Verification items for the finished model (mm, model axes). A direction names the side the tool comes from. Coordinates: 2 decimals unless noted, no trailing zeros. Order: outer loops, then holes, each group sorted by start corner. A loop starts at its lowest first (then second) coordinate and runs counter-clockwise, first axis right, second up. Notation, with made-up numbers: M 16.5,80 L 23.5,80 A23 ccw 23.5,105 Z; hole C 41,46.5 d5. An arc over 180 degrees is marked long. Answer as a JSON object with one key per item and string values. Group by question number.
(1) Cross-section at A-A (z = 0). Enter the section's corners in (x, y), plus the area to 3 significant figures.
(2) Gauge pin test, flat ends, axial feed: pin 1 Ø1 at (y, z) = (-9, 1) entering from -X; pin 2 Ø6 at (x, y) = (4.5, -12) entering from +Z; pin 3 Ø2 at (x, y) = (-1.5, -0.5) entering from +Z. Record the tip position at first contact, or that the pin passes through.
(3) Access from +Z, -Z, +X, -X, +Y, -Y to the whole of each face (thin tool, end or side, straight path). Record for faces 4 (the face through (4.2, 0, 4.2)), 5 (the face through (-2.17, 0.99, 9.76)).
(4) Cross-section at C-C (y = -4.75). Enter the section's corners in (x, z).
(5) Mould release check, pull along Z, two halves, no side actions. Record for faces 1 (the face through (1, -18, 5)), 2 (the face through (-0.59, -7.86, -4.46)), 3 (the face through (-0.75, -8.87, 5.7)): released by +Z, released by -Z, zero draft, split by the parting line, or undercut.
(6) Material ranges on line 1 (Z direction, x = 0, y = -2.5); line 2 (Y direction, x = -7.5, z = 1.25); line 3 (X direction, y = -1, z = 0.25), recorded low to high.
(7) Cross-section at B-B (x = 0). Enter the section's corners in (y, z), plus the area to 3 significant figures.
from build123d import *

# Parameters (mm, degrees)
SKETCH_1_R          = 10
EXTRUDE_1_DEPTH     = 2
SKETCH_2_R          = 5.75
EXTRUDE_2_DEPTH     = 18
CUT_EXTRUDE_1_REACH = 22
SKETCH_3_R          = 4.5
CHAMFER_1_SIZE      = 0.25
FILLET_1_R          = 0.25


with BuildPart() as part:
    # ｽｹｯﾁ1 → ﾎﾞｽ - 押し出し1 (new body)
    with BuildSketch(Plane(origin=(0, 0, 0), x_dir=(1, 0, 0), z_dir=(0, 1, 0))):
        Circle(SKETCH_1_R)
    extrude(amount=EXTRUDE_1_DEPTH)

    # ｽｹｯﾁ2 → ﾎﾞｽ - 押し出し2 (add)
    with BuildSketch(Plane.XZ):
        Circle(SKETCH_2_R)
    extrude(amount=EXTRUDE_2_DEPTH)

    # ｽｹｯﾁ3 → ｶｯﾄ - 押し出し1 (cut, up to next)
    with BuildSketch(Plane(origin=(0, 2, 0), x_dir=(1, 0, 0), z_dir=(0, 1, 0)), mode=Mode.PRIVATE) as cut_extrude_1_sk1:
        Circle(SKETCH_3_R)
    cut_extrude_1_tool1 = extrude(cut_extrude_1_sk1.sketch, amount=-CUT_EXTRUDE_1_REACH, mode=Mode.PRIVATE) & part.part
    add(cut_extrude_1_tool1.solids().sort_by_distance((0, 2, 0))[0], mode=Mode.SUBTRACT)

    # 面取り1
    chamfer_1_edges = [part.edges().sort_by_distance(p)[0] for p in [
        (-10, 0, 0),
        (-10, 2, 0),
    ]]
    chamfer(chamfer_1_edges, length=CHAMFER_1_SIZE)

    # ﾌｨﾚｯﾄ1
    fillet_1_edges = [part.edges().sort_by_distance(p)[0] for p in [
        (-4.5, -18, 0),
        (-4.5, 2, 0),
    ]]
    fillet(fillet_1_edges, radius=FILLET_1_R)


solid = part.part
Taken from the geometry:
{
 "1": {"outline": "M -10,0.25 L -9.75,0 L -5.75,0 L -5.75,-18 L -4.75,-18 A0.25 ccw -4.5,-17.75 L -4.5,1.75 A0.25 ccw -4.75,2 L -9.75,2 L -10,1.75 Z; M 4.5,-17.75 A0.25 ccw 4.75,-18 L 5.75,-18 L 5.75,0 L 9.75,0 L 10,0.25 L 10,1.75 L 9.75,2 L 4.75,2 A0.25 ccw 4.5,1.75 Z", "area": "66.8 mm²"},
 "2": {"pin 1": "stops at x = -5.73", "pin 2": "stops at z = 5.55", "pin 3": "stops at z = 9.96"},
 "3": {"face 4": "-Y", "face 5": "+Y, -Y"},
 "4": {"outline": "C 0,0 d11.5; hole C 0,0 d9"},
 "5": {"face 1": "zero draft", "face 2": "undercut", "face 3": "split by the parting line"},
 "6": {"line 1": "z = -5.75 to -4.5, 4.5 to 5.75", "line 2": "y = 0 to 2", "line 3": "x = -5.74 to -4.49, 4.49 to 5.74"},
 "7": {"outline": "M -18,-5.75 L 0,-5.75 L 0,-9.75 L 0.25,-10 L 1.75,-10 L 2,-9.75 L 2,-4.75 A0.25 ccw 1.75,-4.5 L -17.75,-4.5 A0.25 ccw -18,-4.75 Z; M -18,4.75 A0.25 ccw -17.75,4.5 L 1.75,4.5 A0.25 ccw 2,4.75 L 2,9.75 L 1.75,10 L 0.25,10 L 0,9.75 L 0,5.75 L -18,5.75 Z", "area": "66.8 mm²"}
}
